Geometry check sheet. Reference: drawing and pictorial views, mm from the part's lowest x, y, z. Coordinates: 2 decimals unless noted, no trailing zeros. Loops run counter-clockwise (first coordinate to the right, second up) from the corner with the lowest first, then second, coordinate; pieces in that order, holes last.
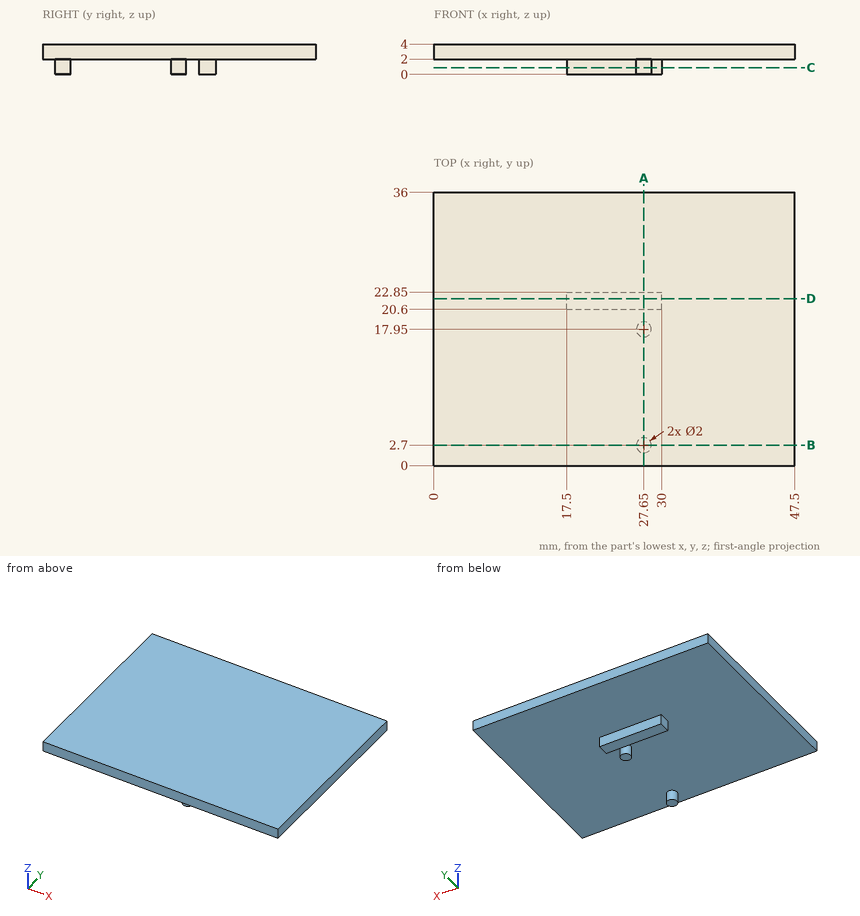
1) Section check B-B on y = 2.7. Record the cut outline in (x, z), and give its area (3 significant figures).
Data:
outline: (0, 2) - (26.65, 2) - (26.65, 0) - (28.65, 0) - (28.65, 2) - (47.5, 2) - (47.5, 4) - (0, 4) - close
area: 99.0 mm2
2) Section check A-A on x = 27.65. Record the cut outline in (y, z), and give its area (3 significant figures).
Data:
outline: (0, 2) - (1.7, 2) - (1.7, 0) - (3.7, 0) - (3.7, 2) - (16.95, 2) - (16.95, 0) - (18.95, 0) - (18.95, 2) - (20.6, 2) - (20.6, 0) - (22.85, 0) - (22.85, 2) - (36, 2) - (36, 4) - (0, 4) - close
area: 84.5 mm2
3) Depth check by flat-ended pin: pin 1 (1.6 mm diameter, centred on y = 22, z = 0.5, fed in from -X); pin 2 (2 mm diameter, centred on x = 25.5, z = 0.5, fed in from +Y); pin 3 (0.6 mm diameter, centred on x = 25, z = 1, fed in from -Y). Enter the tip coordinate at first touch or a pass-through.
Data:
pin 1: stops at x = 17.5
pin 2: stops at y = 22.85
pin 3: stops at y = 20.6
4) Section check D-D on y = 22. Record the cut outline in (x, z), and give its area (3 significant figures).
Data:
outline: (0, 2) - (17.5, 2) - (17.5, 0) - (30, 0) - (30, 2) - (47.5, 2) - (47.5, 4) - (0, 4) - close
area: 120 mm2
5) Material ranges on probe 1 along Z at (x, y) = (11.5, 11); probe 2 along X at (y, z) = (18, 0.8), recorded low to high.
Data:
probe 1: z = 2 to 4
probe 2: x = 26.65 to 28.65
6) Section check C-C on z = 0.9. Record the cut outline in (x, y), and give its area (3 significant figures).
Data:
outline: (17.5, 20.6) - (30, 20.6) - (30, 22.85) - (17.5, 22.85) - close; circle Ø2 at (27.65, 2.7); circle Ø2 at (27.65, 17.95)
area: 34.4 mm2
